Autodesk Inventor part; units mm, degrees
ref_plane "YZ Plane" through (0, 0, 0) normal (1, 0, 0) x (0, 1, 0)
ref_plane "XZ Plane" through (0, 0, 0) normal (0, 1, 0) x (-1, 0, 0)
ref_plane "XY Plane" through (0, 0, 0) normal (0, 0, 1) x (1, 0, 0)
sketch "Эскиз1" plane through (0, 0, 0) normal (0, 1, 0) x (-1, 0, 0)
  line L0 (-44, 145) -> (44, 145)
  line L1 (44, 145) -> (44, -145)
  line L2 (44, -145) -> (-44, -145)
  line L3 (-44, -145) -> (-44, 145)
  line L4 (-44, 145) -> (44, -145) construction
  line L5 (44, 145) -> (-44, -145) construction
  line L6 (44, 0) -> (4, 0)
  circle A0 centre (4, 0) radius 8.5
  point P0 (0, 0)
  dimension "d0" = 88
  dimension "d1" = 290
  dimension "d2" = 40
  dimension "d3" = 17
extrude "Выдавливание1" add sketch "Эскиз1" along normal blind 20
sketch "Эскиз2" plane through (44, 0, 145) normal (1, 0, 0) x (0, 0, -1)
  line L0 (0, 0) -> (290, 0)
  line L1 (290, 0) -> (290, 58)
  line L2 (290, 58) -> (0, 58)
  line L3 (0, 58) -> (0, 0)
  line L4 (0, 58) -> (145, 58)
  line L5 (145, 58) -> (145, 45)
  circle A0 centre (145, 45) radius 5.5
  point P0 (145, 0)
  dimension "d6" = 58
  dimension "d7" = 145
  dimension "d8" = 13
  dimension "d9" = 11
extrude "Выдавливание2" add sketch "Эскиз2" against normal blind 8
properties part number "Угольник-10"
Work out the finished part from the listing and answer in its coordinate system (mm). Give positions to 0.01 mm unless a question says otherwise; leave off trailing zeros. Loops run counter-clockwise (first coordinate to the right, second up) from the corner with the lowest first, then second, coordinate; pieces in that order, holes last. Notation, with made-up numbers: (-4, 25.5) -> (2, 25.5) arc R31 cw to (2, 63.5) -> close; hole circle Ø11 at (15.5, -2). An arc over 180 degrees is marked (long way). Use a Markdown table: item, result. Add a question column.
1) The part is cut by section B-B, the plane y = 45. Determine the outline of the cut face in (x, z).
2) The part is cut by section C-C, the plane z = 110. Determine the outline of the cut face in (x, y).
3) The part is cut by section A-A, the plane z = 0. Determine the outline of the cut face in (x, y).
4) For a pull along Y with two mould halves and no side action, classify faces 1 (the flat face through (5, 20, 2)), 2 (the flat face through (10, 0, 2)), 3 (the flat face through (36, 39, 2)), 4 (the cylindrical face through (40.056, 50.453, 0.716)) as +Y half, -Y half, draft (parallel to the pull), parting line (faces both ways), or undercut.
5) Each of these flat-tipped pins is pushed along its axis until it touches: P1, Ø12, axis at y = 44.5, z = 32, coming from the -X side; P2, Ø1.5, axis at x = 23, z = 102, coming from the +Y side. Where does it stop, or does it pass through?
6) Consider line 1 along Y through (x, z) = (38, 0); line 2 along Z through (x, y) = (-4, 13); line 3 along Z through (x, y) = (42, 45). Determine where each line is inside the solid, lowest interval first.
7) The part is cut by section D-D, the plane y = 29. Determine the outline of the cut face in (x, z).
Reported:
| question | item | result |
|---|---|---|
| 1 | outline | (36, -145) -> (44, -145) -> (44, -5.5) -> (36, -5.5) -> close; (36, 5.5) -> (44, 5.5) -> (44, 145) -> (36, 145) -> close |
| 2 | outline | (-44, 0) -> (44, 0) -> (44, 58) -> (36, 58) -> (36, 20) -> (-44, 20) -> close |
| 3 | outline | (-44, 0) -> (-12.5, 0) -> (-12.5, 20) -> (-44, 20) -> close; (4.5, 0) -> (44, 0) -> (44, 39.5) -> (36, 39.5) -> (36, 20) -> (4.5, 20) -> close; (36, 50.5) -> (44, 50.5) -> (44, 58) -> (36, 58) -> close |
| 4 | face 1 | +Y half |
| 4 | face 2 | -Y half |
| 4 | face 3 | draft |
| 4 | face 4 | undercut |
| 5 | P1 | stops at x = 36 |
| 5 | P2 | stops at y = 20 |
| 6 | line 1 | y = 0 to 39.5, 50.5 to 58 |
| 6 | line 2 | z = -145 to -8.5, 8.5 to 145 |
| 6 | line 3 | z = -145 to -5.5, 5.5 to 145 |
| 7 | outline | (36, -145) -> (44, -145) -> (44, 145) -> (36, 145) -> close |
